```python
from build123d import *

# Parameters (mm, degrees)
BOSS_EXTRUDE1_DEPTH     = 2.5
CUT_EXTRUDE1_DEPTH      = 193.435053979
CUT_EXTRUDE1_DEPTH_BACK = 193.435053979
SKETCH2_W               = 350
SKETCH2_H               = 40


with BuildPart() as part:
    # Sketch1 → Boss-Extrude1 (new, symmetric)
    with BuildSketch(Plane(origin=(0, 0, 0), x_dir=(1, 0, 0), z_dir=(0, 1, 0))):
        Polygon((-80, 0), (80, 0), (80, 75), (0, 175), (-80, 75), align=None)
    extrude(amount=BOSS_EXTRUDE1_DEPTH, both=True)

    # Sketch2 → Cut-Extrude1 (cut, two sides: drawn at the far end of the back side and taken through both)
    with BuildSketch(Plane(origin=(0, 0, 0), x_dir=(1, 0, 0), z_dir=(0, 1, 0)).offset(-CUT_EXTRUDE1_DEPTH_BACK)):
        with Locations((0, 155)):
            Rectangle(SKETCH2_W, SKETCH2_H)
    extrude(amount=CUT_EXTRUDE1_DEPTH + CUT_EXTRUDE1_DEPTH_BACK, mode=Mode.SUBTRACT)


solid = part.part
```
Geometry check sheet. Reference: the model listing, model coordinates, mm. Round coordinates to 2 decimals unless told otherwise and drop trailing zeros. Loops run counter-clockwise (first coordinate to the right, second up) from the corner with the lowest first, then second, coordinate; pieces in that order, holes last. Notation, with made-up numbers: M -38,88.25 L -20,88.25 A32 cw -20,124.25 Z; hole C 12.25,38.5 d3. An arc over 180 degrees is marked long. Return JSON: item names as keys, results as strings. Group by question number.
(1) Section check C-C, the plane z = -120. Enter the section's corners in (x, y).
(2) Scan lines: line 1 along Z through (x, y) = (72, 1.7); line 2 along X through (y, z) = (-0.5, -93); line 3 along Z through (x, y) = (-63, 0.75). Record each from-to range of solid material in increasing order. Write a range as [from, to].
(3) Section check B-B, the plane y = 0.25. Enter the section's corners in (x, z).
(4) Section check A-A, the plane x = 38. Enter the section's corners in (y, z), and give its area (4 significant figures).
Data:
{
 "1": {"outline": "M -44,-2.5 L 44,-2.5 L 44,2.5 L -44,2.5 Z"},
 "2": {"line 1": "[-85, 0]", "line 2": "[-65.6, 65.6]", "line 3": "[-96.25, 0]"},
 "3": {"outline": "M -80,-75 L -32,-135 L 32,-135 L 80,-75 L 80,0 L -80,0 Z"},
 "4": {"outline": "M -2.5,-127.5 L 2.5,-127.5 L 2.5,0 L -2.5,0 Z", "area": "637.5 mm²"}
}
